Source: CAD feature listing. Evaluate the final solid. Frame: model axes, mm. A direction names the side the tool comes from. Round coordinates to 2 decimals unless told otherwise and drop trailing zeros. Loops run counter-clockwise (first coordinate to the right, second up) from the corner with the lowest first, then second, coordinate; pieces in that order, holes last.
Item 1: Section query A-A on y = 38.5. Return loops of the section in (x, z), then the cut area to 3 significant figures.
Item 2: Section query C-C on z = 37. Return loops of the section in (x, y).
Item 3: Access query for faces 1 (the flat face through (26, 25, -39)), 2 (the flat face through (-26, 25, 39)), 3 (the flat face through (-40, 31, -31)). Directions: +Z, -Z, +X, -X, +Y, -Y. A direction counts if a zero-diameter tool reaches every point of the face in a straight line with its end or side. Return the directions, or none.
Item 4: Ray query, L1, parallel to Y at x = 50.5, z = 0; L2, parallel to X at y = 5, z = 0; L3, parallel to X at y = 58, z = 26.5. Return the intervals inside material, ascending.
Item 5: Section query B-B on x = 15.5. Return loops of the section in (y, z).
Item 6: Pull-direction query (X, two-part tool) for faces 4 (the flat face through (-40, 31, 32)), 5 (the flat face through (-1, 25, -1)), 6 (the flat face through (69, 30, -10)), 7 (the flat face through (-39, 0, 10)); classes: released by +X, released by -X, zero draft, split by the parting line, or undercut.
Item 7: First-contact query: P1, Ø10, axis at x = -27, z = 16.5, coming from the -Y side; P2, Ø24, axis at y = 54, z = 1, coming from the +X side; P3, Ø12, axis at x = 55.5, z = -35, coming from the -Y side. Flat tips, straight axial feed; report the tip coordinate or a pass-through.
Item 8: Section query D-D on x = 50. Return loops of the section in (y, z).
```python
from build123d import *

# Parameters (mm, degrees)
SKETCH1_R           = 44
SKETCH1_R_2         = 40
BOSS_EXTRUDE1_DEPTH = 25
SKETCH2_R           = 44
SKETCH2_R_2         = 40
BOSS_EXTRUDE2_DEPTH = 25
SKETCH3_W           = 88
SKETCH3_H           = 88
BOSS_EXTRUDE3_DEPTH = 88
CHAMFER2_SIZE       = 10


with BuildPart() as part:
    # Sketch1 → Boss-Extrude1 (new body)
    with BuildSketch(Plane(origin=(0, 0, 0), x_dir=(1, 0, 0), z_dir=(0, 1, 0))):
        with Locations(Location((0, 0, 0), (0, 0, 270))):
            Circle(SKETCH1_R)
        with Locations(Location((0, 0, 0), (0, 0, 270))):
            Circle(SKETCH1_R_2, mode=Mode.SUBTRACT)
    extrude(amount=BOSS_EXTRUDE1_DEPTH)



with BuildPart() as body_2:
    # Sketch2 → Boss-Extrude2 (new body)
    with BuildSketch(Plane(origin=(44, 0, 0), x_dir=(0, 0, -1), z_dir=(1, 0, 0))):
        with Locations((0, 69)):
            Circle(SKETCH2_R)
        with Locations((0, 69)):
            Circle(SKETCH2_R_2, mode=Mode.SUBTRACT)
    extrude(amount=BOSS_EXTRUDE2_DEPTH)


with BuildPart() as part_1:
    add(part.part)

    add(body_2.part)  # Boss-Extrude3 merges body 2
    # Sketch3 → Boss-Extrude3 (add)
    with BuildSketch(Plane(origin=(0, 25, 0), x_dir=(1, 0, 0), z_dir=(0, 1, 0))):
        Rectangle(SKETCH3_W, SKETCH3_H)
    extrude(amount=BOSS_EXTRUDE3_DEPTH)

    # Chamfer2
    # the kernel refuses this chamfer: 10 mm, written as the material it takes off along each edge
    with BuildSketch(Plane(origin=(-44, 25, 8.9e-08), x_dir=(0.9996219169112968, -0.027495876610586317, 0), z_dir=(0, 0, -1))) as chamfer2_piece_1_section:
        Polygon((CHAMFER2_SIZE * 0.999621916911, -CHAMFER2_SIZE * 0.0274958766106), (-CHAMFER2_SIZE * 0.0274958766106, -CHAMFER2_SIZE * 0.999621916911), (0, 0), align=None)
    chamfer2_piece_1 = extrude(amount=69.716829969, mode=Mode.PRIVATE)
    chamfer2_piece_1 = chamfer2_piece_1 - Plane(origin=(0, 28.58171052, 0), x_dir=(0, 0, 1), z_dir=(0, -1, 0)) * Cylinder(44, 180, mode=Mode.PRIVATE)
    add(chamfer2_piece_1, mode=Mode.SUBTRACT)
    with BuildSketch(Plane(origin=(-44, 25, 69.71682988), x_dir=(0.9996219169112968, -0.027495876610586317, 0), z_dir=(0, 0, -1))) as chamfer2_piece_2_section:
        Polygon((CHAMFER2_SIZE * 0.999621916911, -CHAMFER2_SIZE * 0.0274958766106), (-CHAMFER2_SIZE * 0.0274958766106, -CHAMFER2_SIZE * 0.999621916911), (0, 0), align=None)
    chamfer2_piece_2 = extrude(amount=69.716829791, mode=Mode.PRIVATE)
    chamfer2_piece_2 = chamfer2_piece_2 - Plane(origin=(0, 28.58171052, 0), x_dir=(0, 0, 1), z_dir=(0, -1, 0)) * Cylinder(44, 180, mode=Mode.PRIVATE)
    add(chamfer2_piece_2, mode=Mode.SUBTRACT)
    with BuildSketch(Plane(origin=(44, 25, -1.49e-07), x_dir=(-0.9996219169112968, -0.027495876610586317, 0), z_dir=(0, 0, 1))) as chamfer2_piece_3_section:
        Polygon((CHAMFER2_SIZE * 0.999621916911, -CHAMFER2_SIZE * 0.0274958766106), (-CHAMFER2_SIZE * 0.0274958766106, -CHAMFER2_SIZE * 0.999621916911), (0, 0), align=None)
    chamfer2_piece_3 = extrude(amount=69.716830028, mode=Mode.PRIVATE)
    chamfer2_piece_3 = chamfer2_piece_3 - Plane(origin=(0, 28.146935755, 0), x_dir=(0, 0, 1), z_dir=(0, -1, 0)) * Cylinder(44, 180, mode=Mode.PRIVATE)
    chamfer2_piece_3 = chamfer2_piece_3 - Plane(origin=(40.853064245, 69, 0), x_dir=(0, 0, -1), z_dir=(-1, 0, 0)) * Cylinder(44, 180, mode=Mode.PRIVATE)
    add(chamfer2_piece_3, mode=Mode.SUBTRACT)
    with BuildSketch(Plane(origin=(44, 25, -69.71682988), x_dir=(-0.9996219169112968, -0.027495876610586317, 0), z_dir=(0, 0, 1))) as chamfer2_piece_4_section:
        Polygon((CHAMFER2_SIZE * 0.999621916911, -CHAMFER2_SIZE * 0.0274958766106), (-CHAMFER2_SIZE * 0.0274958766106, -CHAMFER2_SIZE * 0.999621916911), (0, 0), align=None)
    chamfer2_piece_4 = extrude(amount=69.716829731, mode=Mode.PRIVATE)
    chamfer2_piece_4 = chamfer2_piece_4 - Plane(origin=(0, 28.146935758, 0), x_dir=(0, 0, 1), z_dir=(0, -1, 0)) * Cylinder(44, 180, mode=Mode.PRIVATE)
    chamfer2_piece_4 = chamfer2_piece_4 - Plane(origin=(40.853064242, 69, 0), x_dir=(0, 0, -1), z_dir=(-1, 0, 0)) * Cylinder(44, 180, mode=Mode.PRIVATE)
    add(chamfer2_piece_4, mode=Mode.SUBTRACT)
    with BuildSketch(Plane(origin=(-44, 113, 69.71682988), x_dir=(-0.027495876610586317, -0.9996219169112968, 0), z_dir=(0, 0, -1))) as chamfer2_piece_5:
        Polygon((CHAMFER2_SIZE * 0.999621916911, -CHAMFER2_SIZE * 0.0274958766106), (-CHAMFER2_SIZE * 0.0274958766106, -CHAMFER2_SIZE * 0.999621916911), (0, 0), align=None)
    extrude(amount=139.433659759, mode=Mode.SUBTRACT)
    with BuildSketch(Plane(origin=(44, 113, -1.44e-07), x_dir=(-0.9996219169112968, 0.027495876610586317, 0), z_dir=(0, 0, 1))) as chamfer2_piece_6_section:
        Polygon((CHAMFER2_SIZE * 0.999621916911, CHAMFER2_SIZE * 0.0274958766106), (-CHAMFER2_SIZE * 0.0274958766106, CHAMFER2_SIZE * 0.999621916911), (0, 0), align=None)
    chamfer2_piece_6 = extrude(amount=69.716830024, mode=Mode.PRIVATE)
    chamfer2_piece_6 = chamfer2_piece_6 - Plane(origin=(40.41828948, 69, 0), x_dir=(0, 0, -1), z_dir=(-1, 0, 0)) * Cylinder(44, 180, mode=Mode.PRIVATE)
    add(chamfer2_piece_6, mode=Mode.SUBTRACT)
    with BuildSketch(Plane(origin=(44, 113, -69.71682988), x_dir=(-0.9996219169112968, 0.027495876610586317, 0), z_dir=(0, 0, 1))) as chamfer2_piece_7_section:
        Polygon((CHAMFER2_SIZE * 0.999621916911, CHAMFER2_SIZE * 0.0274958766106), (-CHAMFER2_SIZE * 0.0274958766106, CHAMFER2_SIZE * 0.999621916911), (0, 0), align=None)
    chamfer2_piece_7 = extrude(amount=69.716829736, mode=Mode.PRIVATE)
    chamfer2_piece_7 = chamfer2_piece_7 - Plane(origin=(40.41828948, 69, 0), x_dir=(0, 0, -1), z_dir=(-1, 0, 0)) * Cylinder(44, 180, mode=Mode.PRIVATE)
    add(chamfer2_piece_7, mode=Mode.SUBTRACT)


solid = part_1.part
```
Data:
1. outline: (-44, -44) - (44, -44) - (44, -31.71) - (69, -31.71) - (69, -25.88) - (44, -25.88) - (44, 25.88) - (69, 25.88) - (69, 31.71) - (44, 31.71) - (44, 44) - (-44, 44) - close
1. area: 8,040 mm2
2. outline: (-44, 35) - (-34, 25) - (-23.81, 25) - (-23.81, 0) - (-15.2, 0) - (-15.2, 25) - (15.2, 25) - (15.2, 0) - (23.81, 0) - (23.81, 25) - (34, 25) - (44, 35) - (44, 45.19) - (69, 45.19) - (69, 53.8) - (44, 53.8) - (44, 84.2) - (69, 84.2) - (69, 92.81) - (44, 92.81) - (44, 103) - (34, 113) - (-34, 113) - (-44, 103) - close
3. face 1: -Z, +X, -Y
3. face 2: +Z, -X, -Y
3. face 3: -Z, -X, -Y
4. L1: y = 25 to 29, 109 to 113
4. L2: x = -44 to -40, 40 to 44
4. L3: x = -44 to 44
5. outline: (0, -41.18) - (25, -41.18) - (25, -44) - (113, -44) - (113, 44) - (25, 44) - (25, 41.18) - (0, 41.18) - (0, 36.87) - (25, 36.87) - (25, -36.87) - (0, -36.87) - close
6. face 4: released by -X
6. face 5: undercut
6. face 6: released by +X
6. face 7: zero draft
7. P1: stops at y = 25
7. P2: stops at x = 44
7. P3: stops at y = 35.91
8. outline: circle Ø88 at (69, 0); hole circle Ø80 at (69, 0)
